Design review of the part built by this model. Coordinates are the model's own, in mm. A direction names the side the tool comes from. Coordinates: 2 decimals unless noted, no trailing zeros. Write each loop counter-clockwise with the first axis right and the second up, starting at its lowest first coordinate (ties: lowest second). Pieces come first, ordered by that corner, then holes.
Q1. Mouldability with a two-part tool opening along X and no side actions: class faces 1 (the flat face through (3, -3, 3.298)), 2 (the flat face through (3, 0, -3.452)), 3 (the flat face through (6, 0, -1)), 4 (the flat face through (-4, 4, 2.798)) as pulls with the +X half, pulls with the -X half, needs draft (parallel to the pull), parting line crosses it, or undercut.
Q2. Take a section at B-B (z = 2.5). Give the boundary of the cut face in (x, y), and give its area (3 significant figures).
Q3. For probe 1 along X at (y, z) = (-2, -3); probe 2 along Z at (x, y) = (3, -4.25); probe 3 along Z at (x, y) = (0.75, 4.75), list the stretches that pass through material, from the lowest coordinate up.
Q4. Take a section at A-A (z = -2.75). Give the boundary of the cut face in (x, y) (3 decimals), and give its area (3 significant figures).
Q5. Insertion check: pin 1 (0.5 mm diameter, centred on x = 3.5, y = 0.5, fed in from +Z); pin 2 (2 mm diameter, centred on x = 0.5, y = -2.5, fed in from -Z); pin 3 (1.1 mm diameter, centred on x = 3.5, y = -4, fed in from +Z). Each pin has a flat end and moves straight along its axis. Give the tip position at first contact, or say it passes through.
Q6. Machinability: for faces 5 (the flat face through (-4.275, 0, -1)), 6 (the flat face through (-6, 0, -1)), 7 (the flat face through (4, -4, 2.798)), which of the approach directions +Z, -Z, +X, -X, +Y, -Y give a long, thin tool a straight path to every point of the face, cutting with its end or side? Answer none if there is none.
```python
from build123d import *

# Parameters (mm, degrees)
F1_DEPTH = 6
F2_R     = 0.5
F3_R     = 0.5
F5_DEPTH = 0.5
F5_TAPER = 30
F6_R     = 0.5


with BuildPart() as f1:
    # F0 (on Front) → F1 (new body, symmetric)
    with BuildSketch(Plane.XZ):
        Polygon((6, -4.5523648744), (6, 2.7976351256), (-6, 2.7976351256), (-6, -4.5523648744), (-2.2, -4.5523648744), (-2.2, -3.4523648744), (-4.275, -3.4523648744), (-4.275, 1.7976351256), (4.225, 1.7976351256), (4.225, -3.4523648744), (2.2, -3.4523648744), (2.2, -4.5523648744), align=None)
    extrude(amount=F1_DEPTH, both=True)

    # F2
    f2_edges = [f1.edges().sort_by_distance(p)[0] for p in [
        (-2.2, 0, -4.552365),
        (2.2, 0, -4.552365),
        (-2.2, 0, -3.452365),
        (2.2, 0, -3.452365),
    ]]
    fillet(f2_edges, radius=F2_R)

    # F3
    f3_edges = [f1.edges().sort_by_distance(p)[0] for p in [
        (6, 0, -4.552365),
        (6, 6, -0.877365),
        (6, 0, 2.797635),
        (6, -6, -0.877365),
        (0, 6, 2.797635),
        (-6, 0, 2.797635),
        (0, -6, 2.797635),
        (-6, 6, -0.877365),
        (-6, 0, -4.552365),
        (-6, -6, -0.877365),
    ]]
    fillet(f3_edges, radius=F3_R)

    # F4 (on face) → F5 (join)
    with BuildSketch(Plane.XY.offset(2.7976351256)):
        Polygon((-0.8431457505, 4.5), (0.1568542495, 5.5), (-1.2573593129, 5.5), (-2.2573593129, 4.5), align=None)
        Polygon((-4.5, 0.8431457505), (-0.8431457505, 4.5), (-2.2573593129, 4.5), (-4.5, 2.2573593129), align=None)
        Polygon((-5.5, 1.2573593129), (-5.5, -0.1568542495), (-4.5, 0.8431457505), (-4.5, 2.2573593129), align=None)
        Polygon((-0.1568542495, -5.5), (5.5, -5.5), (5.5, 0.1568542495), (4.5, -0.8431457505), (4.5, -2.2573593129), (4.5, -4.5), (2.2573593129, -4.5), (0.8431457505, -4.5), align=None)
        Polygon((-2.2573593129, 4.5), (-1.2573593129, 5.5), (-5.5, 5.5), (-5.5, 1.2573593129), (-4.5, 2.2573593129), (-4.5, 4.5), align=None)
        Polygon((4.5, -2.2573593129), (4.5, -0.8431457505), (0.8431457505, -4.5), (2.2573593129, -4.5), align=None)
    extrude(amount=F5_DEPTH, taper=F5_TAPER)

    # F6
    f6_edges = [f1.edges().sort_by_distance(p)[0] for p in [
        (-4.275, 0, 1.797635),
        (4.225, 0, 1.797635),
        (-4.275, 0, -3.452365),
        (4.225, 0, -3.452365),
    ]]
    fillet(f6_edges, radius=F6_R)


solid = f1.part
```
Response:
1. face 1: needs draft
1. face 2: undercut
1. face 3: pulls with the +X half
1. face 4: undercut
2. outline: (-5.96, -5.5) arc R0.46 ccw to (-5.5, -5.96) - (5.5, -5.96) arc R0.46 ccw to (5.96, -5.5) - (5.96, 5.5) arc R0.46 ccw to (5.5, 5.96) - (-5.5, 5.96) arc R0.46 ccw to (-5.96, 5.5) - close
2. area: 142 mm2
3. probe 1: x = -6 to -4.27, 4.22 to 6
3. probe 2: z = -4.55 to -3.45, 1.8 to 2.8
3. probe 3: z = 1.8 to 2.8
4. outline: (-6, -5.5) arc R0.5 ccw to (-5.5, -6) - (-4.275, -6) - (-4.275, 6) - (-5.5, 6) arc R0.5 ccw to (-6, 5.5) - close; (4.225, -6) - (5.5, -6) arc R0.5 ccw to (6, -5.5) - (6, 5.5) arc R0.5 ccw to (5.5, 6) - (4.225, 6) - close
4. area: 41.8 mm2
5. pin 1: stops at z = 2.8
5. pin 2: stops at z = 1.8
5. pin 3: stops at z = 2.88
6. face 5: +Y, -Y
6. face 6: +Z, -Z, -X, +Y, -Y
6. face 7: +Z
